Input: dimensioned drawing with shaded views. Units: mm. Origin: part minimum x, y, z. A direction names the side the tool comes from. Give positions to 0.01 mm unless a question says otherwise; leave off trailing zeros. Loops run counter-clockwise (first coordinate to the right, second up) from the corner with the lowest first, then second, coordinate; pieces in that order, holes last.
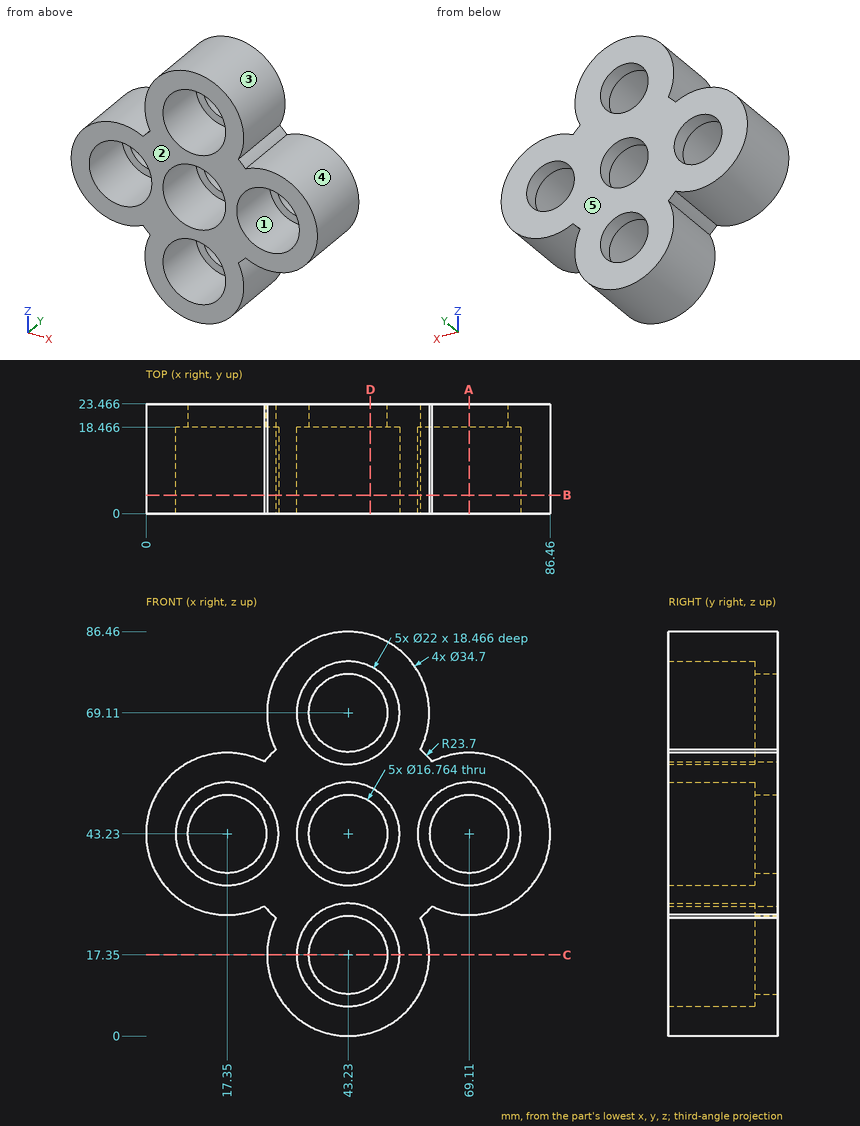
(1) Section C-C, the plane z = 17.35. Return the cut outline in (x, y), then the cut area to 3 significant figures.
A:
outline: (25.88, 0) - (32.23, 0) - (32.23, 18.47) - (34.85, 18.47) - (34.85, 23.47) - (25.88, 23.47) - close; (51.61, 18.47) - (54.23, 18.47) - (54.23, 0) - (60.58, 0) - (60.58, 23.47) - (51.61, 23.47) - close
area: 324 mm2
(2) Reachability of the marked faces 1 and 2 from +Z, -Z, +X, -X, +Y, -Y: full face, straight path, thin tool, end or side. Return the list, or none.
A:
face 1: -Y
face 2: +Z, -Z, +X, -X, -Y
(3) Mould query, pull axis X, two halves, no side actions, for the marked faces 3, 4 and 5. Classes: pulls with the +X half, pulls with the -X half, needs draft (parallel to the pull), parting line crosses it, or undercut.
A:
face 3: parting line crosses it
face 4: undercut
face 5: needs draft
(4) Section D-D, the plane x = 48. Return the cut outline in (y, z).
A:
outline: (0, 0.67) - (23.47, 0.67) - (23.47, 10.46) - (18.47, 10.46) - (18.47, 7.44) - (0, 7.44) - close; (0, 27.26) - (18.47, 27.26) - (18.47, 24.24) - (23.47, 24.24) - (23.47, 36.34) - (18.47, 36.34) - (18.47, 33.32) - (0, 33.32) - close; (0, 53.14) - (18.47, 53.14) - (18.47, 50.12) - (23.47, 50.12) - (23.47, 62.22) - (18.47, 62.22) - (18.47, 59.2) - (0, 59.2) - close; (0, 79.02) - (18.47, 79.02) - (18.47, 76) - (23.47, 76) - (23.47, 85.79) - (0, 85.79) - close
(5) Section A-A, the plane x = 69.11. Return the cut outline in (y, z), then the cut area to 3 significant figures.
A:
outline: (0, 25.88) - (23.47, 25.88) - (23.47, 34.85) - (18.47, 34.85) - (18.47, 32.23) - (0, 32.23) - close; (0, 54.23) - (18.47, 54.23) - (18.47, 51.61) - (23.47, 51.61) - (23.47, 60.58) - (0, 60.58) - close
area: 324 mm2
(6) First-contact query: pin 1 (2 mm diameter, centred on x = 61.5, z = 39, fed in from -Y); pin 2 (10 mm diameter, centred on x = 70, y = 9, fed in from +Z); pin 3 (1 mm diameter, centred on y = 5, z = 18.5, fed in from +X). Flat tips, straight axial feed; report the tip coordinate or a pass-through.
A:
pin 1: stops at y = 18.47
pin 2: stops at z = 60.58
pin 3: stops at x = 60.57
(7) Ray query, line 1 along Z through (x, y) = (43.23, 22); line 2 along X through (y, z) = (1.5, 51.5); line 3 along Z through (x, y) = (18, 19.25). Return the intervals inside material, ascending.
A:
line 1: z = 0 to 8.97, 25.73 to 34.85, 51.61 to 60.73, 77.49 to 86.46
line 2: x = 2.1 to 10.1, 24.6 to 35.98, 50.48 to 61.86, 76.36 to 84.36
line 3: z = 25.89 to 34.87, 51.59 to 60.57
(8) Section B-B, the plane y = 4. Return the cut outline in (x, z) (3 decimals), then the cut area to 3 significant figures.
A:
outline: (25.254, 27.785) arc R23.7 ccw to (27.785, 25.254) arc R17.35 ccw (long way) to (58.675, 25.254) arc R23.7 ccw to (61.206, 27.785) arc R17.35 ccw (long way) to (61.206, 58.675) arc R23.7 ccw to (58.675, 61.206) arc R17.35 ccw (long way) to (27.785, 61.206) arc R23.7 ccw to (25.254, 58.675) arc R17.35 ccw (long way) to start; hole circle Ø22 at (17.35, 43.23); hole circle Ø22 at (43.23, 17.35); hole circle Ø22 at (43.23, 43.23); hole circle Ø22 at (43.23, 69.11); hole circle Ø22 at (69.11, 43.23)
area: 2,330 mm2
